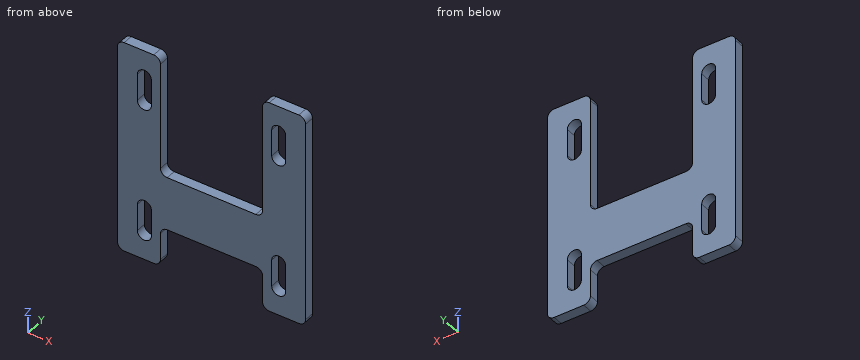
Autodesk Inventor part; units mm, degrees
ref_plane "YZ Plane" through (0, 0, 0) normal (1, 0, 0) x (0, 1, 0)
ref_plane "XZ Plane" through (0, 0, 0) normal (0, 1, 0) x (-1, 0, 0)
ref_plane "XY Plane" through (0, 0, 0) normal (0, 0, 1) x (1, 0, 0)
sketch "Sketch1" plane through (0, 0, 0) normal (0, 1, 0) x (-1, 0, 0)
  line L0 (0, 0) -> (20.32, 0)
  line L1 (0, 101.6) -> (0, 0)
  line L2 (44.45, 44.45) -> (20.32, 44.45)
  line L3 (20.32, 44.45) -> (20.32, 101.6)
  line L4 (44.45, 44.45) -> (44.45, 19.05)
  line L5 (20.32, 101.6) -> (0, 101.6)
  line L6 (16.002, 88.9) -> (16.002, 76.2)
  line L7 (9.398, 76.2) -> (9.398, 88.9)
  arc A0 (16.002, 88.9) -> (9.398, 88.9) centre (12.7, 88.9) ccw
  arc A1 (9.398, 76.2) -> (16.002, 76.2) centre (12.7, 76.2) ccw
  line L8 (16.002, 25.4) -> (16.002, 12.7)
  line L9 (9.398, 12.7) -> (9.398, 25.4)
  arc A2 (16.002, 25.4) -> (9.398, 25.4) centre (12.7, 25.4) ccw
  arc A3 (9.398, 12.7) -> (16.002, 12.7) centre (12.7, 12.7) ccw
  line L10 (44.45, 19.05) -> (20.32, 19.05)
  line L11 (20.32, 19.05) -> (20.32, 0)
  dimension "d1" = 101.6
  dimension "d8" = 44.45
  dimension "d11" = 6.604
  dimension "d14" = 12.7
  dimension "d15" = 12.7
  dimension "d18" = 12.7
  dimension "d19" = 20.32
  dimension "d21" = 31.75
  dimension "d23" = 25.4
  dimension "d24" = 19.05
  dimension "d25" = 63.5
  dimension "d26" = 6.604
extrude "Extrusion1" add sketch "Sketch1" against normal blind 4.7625
fillet "Fillet1" radius 3.175 6 edges at (-20.32, -2.3813, 44.45) (-20.32, -2.3813, 101.6) (0, -2.3813, 101.6) (0, -2.3813, 0) (-20.32, -2.3813, 0) (-20.32, -2.3813, 19.05)
mirror "Mirror2" about plane through (-44.45, 0, 44.45) normal (-1, 0, 0)
equation "\"d26\" = d11"
properties part number "torchMount_back"
Geometry check sheet. Reference: the model listing, model coordinates, mm. Coordinates: 2 decimals unless noted, no trailing zeros. Order: outer loops, then holes, each group sorted by start corner. A loop starts at its lowest first (then second) coordinate and runs counter-clockwise, first axis right, second up.
Item 1: Section check D-D (z = 46). Enter the section's corners in (x, y), plus the area to 3 significant figures.
Item 2: Section check A-A (z = 68). Enter the section's corners in (x, y), plus the area to 3 significant figures.
Item 3: Scan lines: line 1 along X through (y, z) = (-3.55, 86.5); line 2 along X through (y, z) = (-2.95, 68.5); line 3 along X through (y, z) = (-3.85, 10). Record each from-to range of solid material in increasing order.
Item 4: Section check B-B (y = -3.2). Count the separate pieces of the cut face and the enclosed holes in it, plus the area to 3 significant figures.
Item 5: Section check C-C (x = -32). Enter the section's corners in (y, z).
Item 6: Depth check by flat-ended pin: pin 1 (1.4 mm diameter, centred on x = -43, y = -2.5, fed in from +Z); pin 2 (2.5 mm diameter, centred on x = -48.5, y = -2, fed in from -Z). Enter the tip coordinate at first touch or a pass-through.
Check sheet entries:
1. outline: (-88.9, -4.76) - (-68.13, -4.76) - (-68.13, 0) - (-88.9, 0) - close; (-20.77, -4.76) - (0, -4.76) - (0, 0) - (-20.77, 0) - close
1. area: 198 mm2
2. outline: (-88.9, -4.76) - (-68.58, -4.76) - (-68.58, 0) - (-88.9, 0) - close; (-20.32, -4.76) - (0, -4.76) - (0, 0) - (-20.32, 0) - close
2. area: 194 mm2
3. line 1: x = -88.9 to -79.5, -72.9 to -68.58, -20.32 to -16, -9.4 to 0
3. line 2: x = -88.9 to -68.58, -20.32 to 0
3. line 3: x = -88.9 to -78.1, -74.3 to -68.58, -20.32 to -14.6, -10.8 to 0
4. separate pieces: 1
4. enclosed holes: 4
4. area: 4,870 mm2
5. outline: (-4.76, 19.05) - (0, 19.05) - (0, 44.45) - (-4.76, 44.45) - close
6. pin 1: stops at z = 44.45
6. pin 2: stops at z = 19.05
